Read the model definition and answer for the solid it produces. Units are mm, in the model's axes. Give positions to 0.01 mm unless a question says otherwise; leave off trailing zeros. Loops run counter-clockwise (first coordinate to the right, second up) from the corner with the lowest first, then second, coordinate; pieces in that order, holes last. Notation, with made-up numbers: (0, 29.25) - (22, 29.25) arc R18 cw to (22, 61.25) - close; hole circle Ø7 at (11, 26). An arc over 180 degrees is marked (long way). Write item = value, one per line.
```python
from build123d import *

# Parameters (mm, degrees)
SKETCH1_W                                        = 50.8
SKETCH1_H                                        = 50.8
BOSS_EXTRUDE1_DEPTH                              = 7.26
CBORE_FOR_M5_SBHCS1_D                            = 5.5
CBORE_FOR_M5_SBHCS1_CBORE_D                      = 10.5
CBORE_FOR_M5_SBHCS1_CBORE_DEPTH                  = 2.75
CBORE_FOR_1_4_SOCKET_HEAD_CAP_SCREW1_D           = 6.7564
CBORE_FOR_1_4_SOCKET_HEAD_CAP_SCREW1_CBORE_D     = 11.1125
CBORE_FOR_1_4_SOCKET_HEAD_CAP_SCREW1_CBORE_DEPTH = 6.35
SKETCH6_W                                        = 50.8
SKETCH6_H                                        = 14.52
BOSS_EXTRUDE2_DEPTH                              = 100


with BuildPart() as part:
    # Sketch1 → Boss-Extrude1 (new, symmetric)
    with BuildSketch(Plane(origin=(0, 0, 0), x_dir=(1, 0, 0), z_dir=(0, 1, 0))):
        Rectangle(SKETCH1_W, SKETCH1_H)
    extrude(amount=BOSS_EXTRUDE1_DEPTH, both=True)

    # CBORE for M5 SBHCS1 (through all)
    with Locations(Plane(origin=(0, 7.26, 0), x_dir=(1, 0, 0), z_dir=(0, 1, 0))):
        with Locations((-15, 19), (-15, -19), (15, -19), (15, 19)):
            CounterBoreHole(CBORE_FOR_M5_SBHCS1_D / 2, CBORE_FOR_M5_SBHCS1_CBORE_D / 2, CBORE_FOR_M5_SBHCS1_CBORE_DEPTH)

    # CBORE for 1/4 Socket Head Cap Screw1 (through all)
    with Locations(Plane.XZ.offset(7.26)):
        with Locations((0, 0)):
            CounterBoreHole(CBORE_FOR_1_4_SOCKET_HEAD_CAP_SCREW1_D / 2, CBORE_FOR_1_4_SOCKET_HEAD_CAP_SCREW1_CBORE_D / 2, CBORE_FOR_1_4_SOCKET_HEAD_CAP_SCREW1_CBORE_DEPTH)

    # Sketch6 → Boss-Extrude2 (add)
    with BuildSketch(Plane.ZY.offset(25.4)):
        Rectangle(SKETCH6_W, SKETCH6_H)
    extrude(amount=BOSS_EXTRUDE2_DEPTH)


solid = part.part
```
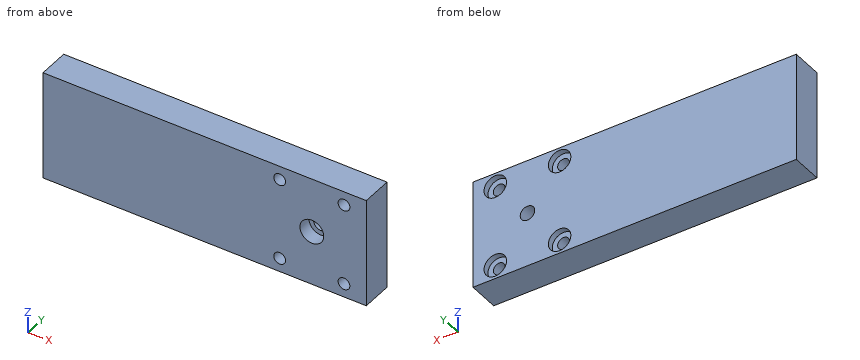
1) Find the intervals of material crossed by probe 1 along X at (y, z) = (-0.75, 19); probe 2 along Z at (x, y) = (15, 5.9); probe 3 along X at (y, z) = (5.55, 19), in increasing order.
Output:
probe_1 = -125.4 to -17.75, -12.25 to 12.25, 17.75 to 25.4
probe_2 = -25.4 to -24.25, -13.75 to 13.75, 24.25 to 25.4
probe_3 = -125.4 to -20.25, -9.75 to 9.75, 20.25 to 25.4
2) Each of these flat-tipped pins is pushed along its axis until it touches: P1, Ø5.5, axis at x = 2.5, z = 0, coming from the -Y side; P2, Ø5, axis at x = 16.5, z = 16.5, coming from the +Y side; P3, Ø9, axis at x = -15, z = 19, coming from the +Y side. Where does it stop, or does it pass through?
Output:
P1 = -0.91
P2 = 7.26
P3 = 4.51
3) A cutting plane is placed at B-B on z = -19. Determine the outline of the cut face in (x, y), then the cut area to 3 significant figures.
Output:
outline = (-125.4, -7.26) - (-17.75, -7.26) - (-17.75, 4.51) - (-20.25, 4.51) - (-20.25, 7.26) - (-125.4, 7.26) - close; (-12.25, -7.26) - (12.25, -7.26) - (12.25, 4.51) - (9.75, 4.51) - (9.75, 7.26) - (-9.75, 7.26) - (-9.75, 4.51) - (-12.25, 4.51) - close; (17.75, -7.26) - (25.4, -7.26) - (25.4, 7.26) - (20.25, 7.26) - (20.25, 4.51) - (17.75, 4.51) - close
area = 2,000 mm²
4) A cutting plane is placed at C-C on y = -3. Determine the outline of the cut face in (x, z), then the cut area to 3 significant figures.
Output:
outline = (-125.4, -25.4) - (25.4, -25.4) - (25.4, 25.4) - (-125.4, 25.4) - close; hole circle Ø5.5 at (-15, -19); hole circle Ø5.5 at (-15, 19); hole circle Ø11.11 at (0, 0); hole circle Ø5.5 at (15, -19); hole circle Ø5.5 at (15, 19)
area = 7,470 mm²
5) A cutting plane is placed at A-A on x = 0. Determine the outline of the cut face in (y, z).
Output:
outline = (-7.26, -25.4) - (7.26, -25.4) - (7.26, -3.38) - (-0.91, -3.38) - (-0.91, -5.56) - (-7.26, -5.56) - close; (-7.26, 5.56) - (-0.91, 5.56) - (-0.91, 3.38) - (7.26, 3.38) - (7.26, 25.4) - (-7.26, 25.4) - close
